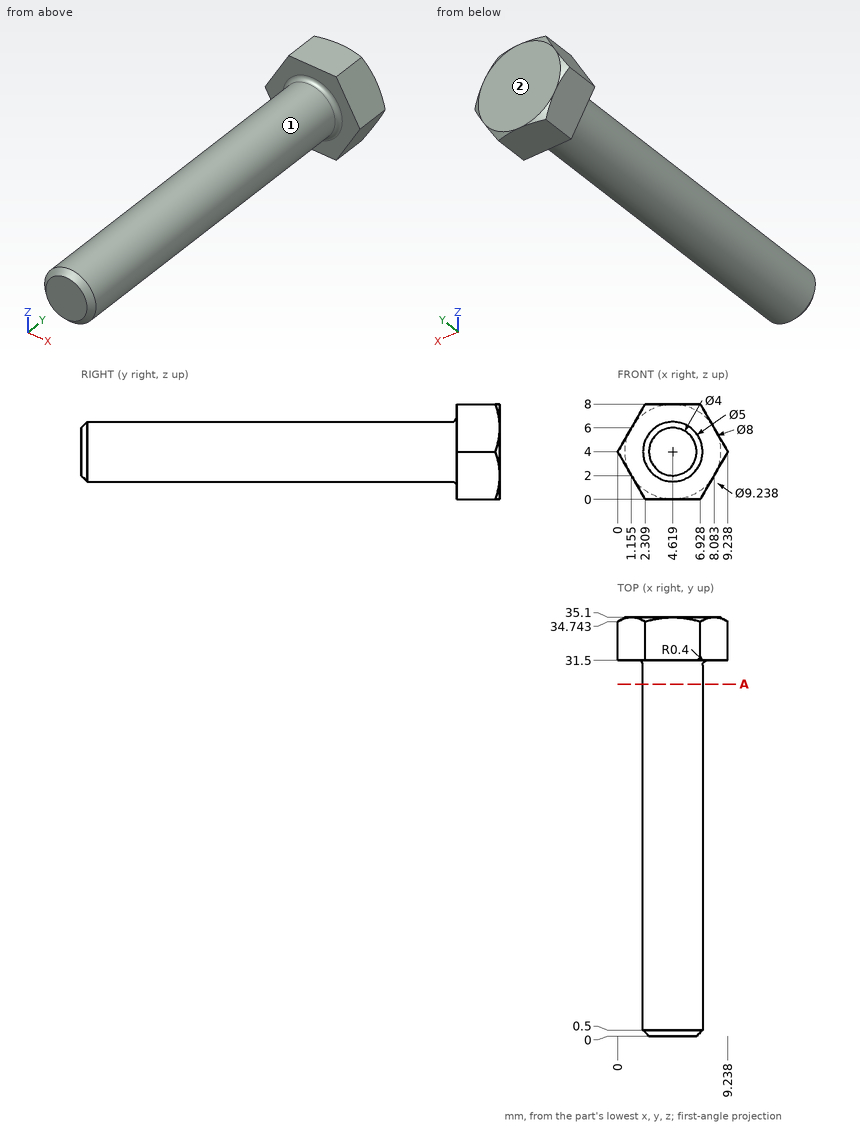
Input: dimensioned drawing with shaded views. Units: mm. Origin: part minimum x, y, z. A direction names the side the tool comes from. Coordinates: 2 decimals unless noted, no trailing zeros. Loops run counter-clockwise (first coordinate to the right, second up) from the corner with the lowest first, then second, coordinate; pieces in that order, holes last. Notation, with made-up numbers: M 20.5,54 L 62.5,54 A15 cw 62.5,67 Z; hole C 62,12 d11. An arc over 180 degrees is marked long. Use a Markdown table: item, result. Add a question column.
1) Set-up query: the marked faces 1 and 2. Return all of +Z, -Z, +X, -X, +Y, -Y with unobstructed straight access to the full face (end or side cutting, diameter ignored); none if empty.
2) Pin query (flat end, axial travel): P1, Ø4, axis at x = 4, y = 17.5, coming from the -Z side; P2, Ø1.5, axis at x = 3.5, y = 9.5, coming from the +Z side; P3, Ø4, axis at y = 4, z = 4.5, coming from the -X side. Return the tip coordinate at first contact, or that it passes through.
3) Section A-A, the plane y = 29.5. Return the cut outline in (x, z).
4) Line query: L1, parallel to Y at x = 6.75, z = 7; L2, parallel to X at y = 12.5, z = 5.5; L3, parallel to Z at x = 4.75, y = 26. Output: solid intervals per line, ascending. Write a range as from..to.
Answer below:
| question | item | result |
|---|---|---|
| 1 | face 1 | -Y |
| 1 | face 2 | +Z, -Z, +X, -X, +Y |
| 2 | P1 | z = 1.5 |
| 2 | P2 | z = 6.47 |
| 2 | P3 | x = 2.12 |
| 3 | outline | C 4.62,4 d5 |
| 4 | L1 | 31.5..35.1 |
| 4 | L2 | 2.62..6.62 |
| 4 | L3 | 1.5..6.5 |
